Here's the drawing with two shaded views (mm, measured from the low corner). I have some questions. A direction names the side the tool comes from. Coordinates: 2 decimals unless noted, no trailing zeros. Loops run counter-clockwise (first coordinate to the right, second up) from the corner with the lowest first, then second, coordinate; pieces in that order, holes last. Notation, with made-up numbers: (83, -29) - (96, -29) arc R12 ccw to (96, -15) - close; hole circle Ø10 at (13.5, -37.5). An arc over 180 degrees is marked (long way). Use a Markdown table: item, result.
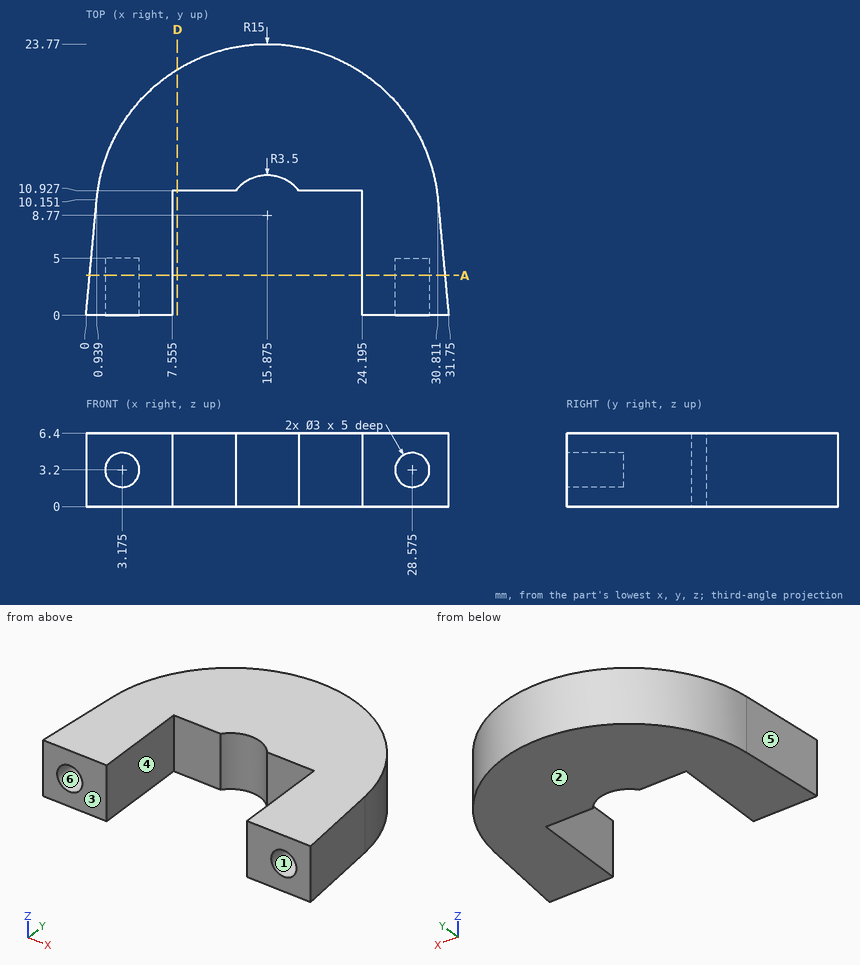
Q1. I want a section at A-A, the plane y = 3.5. Write out the boundary of the cut face in (x, z) (1 decimal).
Check values:
| item | result |
|---|---|
| outline | (0.3, 0) - (7.6, 0) - (7.6, 6.4) - (0.3, 6.4) - close; (24.2, 0) - (31.4, 0) - (31.4, 6.4) - (24.2, 6.4) - close; hole circle Ø3 at (3.2, 3.2); hole circle Ø3 at (28.6, 3.2) |
Q2. Please list where these lines run through material, in increasing order: L1, parallel to X at y = 7, z = 1.5 (1 decimal); L2, parallel to X at y = 11.5, z = 4 (1 decimal); L3, parallel to Y at x = 16, z = 5. Write a range as from..to.
Check values:
| item | result |
|---|---|
| L1 | 0.6..7.6, 24.2..31.1 |
| L2 | 1.1..13.7, 18.1..30.6 |
| L3 | 12.27..23.77 |
Q3. If we mould it in two halves opening along Z, with no side actions, what happens to the marked faces 1, 2 and 3? For each: pulls with the +Z half, pulls with the -Z half, needs draft (parallel to the pull), parting line crosses it, or undercut.
Check values:
| item | result |
|---|---|
| face 1 | undercut |
| face 2 | pulls with the -Z half |
| face 3 | needs draft |
Q4. Which directions (+Z, -Z, +X, -X, +Y, -Y) give clear straight access to the entire face, cutting with the end or side of a thin tool? Please do the marked faces 4, 5 and 6.
Check values:
| item | result |
|---|---|
| face 4 | +Z, -Z, -Y |
| face 5 | +Z, -Z, -X, +Y |
| face 6 | -Y |
Q5. Will these pins go through, and if not, where does the flat tip stop? P1, Ø1.9, axis at y = 3, z = 2.5, coming from the -X side; P2, Ø2.5, axis at x = 3.175, z = 3.2, coming from the -Y side; P3, Ø3, axis at x = 4, z = 4.5, coming from the +Y side.
Check values:
| item | result |
|---|---|
| P1 | x = 0.19 |
| P2 | y = 5 |
| P3 | y = 19.6 |
Q6. I want a section at D-D, the plane x = 8. Write out the boundary of the cut face in (y, z), then the cut area to 3 significant figures.
Check values:
| item | result |
|---|---|
| outline | (10.93, 0) - (21.54, 0) - (21.54, 6.4) - (10.93, 6.4) - close |
| area | 67.9 mm^2 |
